The listing builds one solid part. Answer for the finished solid, in the listing's coordinates (mm). Round coordinates to 2 decimals unless told otherwise and drop trailing zeros. Order: outer loops, then holes, each group sorted by start corner. A loop starts at its lowest first (then second) coordinate and runs counter-clockwise, first axis right, second up. Notation, with made-up numbers: M 61.5,48.5 L 76.5,48.5 A10 cw 76.5,58.5 Z; hole C 1,68.5 d3. An arc over 180 degrees is marked long. Write item = value, one per line. Start each with the question number.
(1) Straight lines are drawn through the part: probe 1 along X at (y, z) = (-0.9, 0); probe 2 along X at (y, z) = (-0.65, -30); probe 3 along Y at (x, z) = (-60.6, 0). For each, find the intervals that lie inside material, in ascending order. Write a range as from..to.
(2) A cutting plane is placed at A-A, the plane z = 0. Count the separate pieces of the cut face and the enclosed holes in it, and give its area (3 significant figures).
(3) A cutting plane is placed at B-B, the plane x = -143. Determine the outline of the cut face in (y, z).
(4) Each of these flat-tipped pins is pushed along its axis until it touches: pin 1 (1 mm diameter, centred on x = -60.5, z = 47.5, fed in from -Y); pin 2 (4 mm diameter, centred on y = -8, z = 11, fed in from +X); pin 3 (3.5 mm diameter, centred on x = -16.5, z = -59.5, fed in from -Y). Where does it stop, or does it pass through?
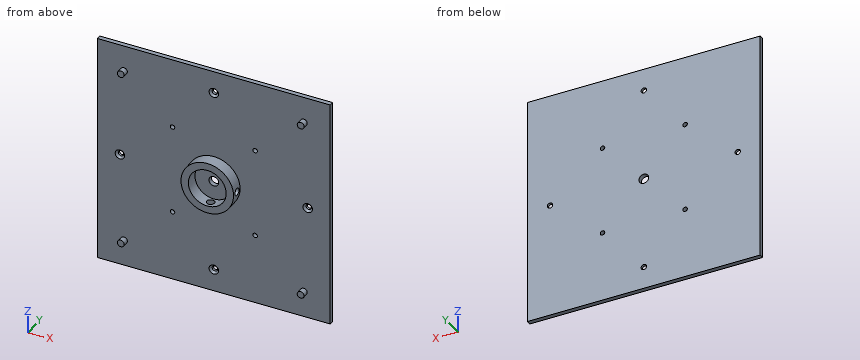
from build123d import *

# Parameters (mm, degrees)
SKETCH10_W                                     = 155
SKETCH10_H                                     = 155
BOSS_EXTRUDE3_DEPTH                            = 3
SKETCH11_R                                     = 17.5
SKETCH11_R_2                                   = 12.59
BOSS_EXTRUDE4_DEPTH                            = 8.4
SKETCH11_4_R                                   = 2.3
BOSS_EXTRUDE6_DEPTH                            = 4
SKETCH12_R                                     = 2.55
CUT_EXTRUDE1_DEPTH                             = 37
SKETCH14_R                                     = 2.55
CUT_EXTRUDE2_DEPTH                             = 75
SKETCH15_R                                     = 1.5
SKETCH15_R_2                                   = 3.25
CUT_EXTRUDE3_DEPTH                             = 95
CSK_FOR_M3_FLAT_HEAD_MACHINE_SCREW1_AT_2_COUNT = 2
CSK_FOR_M3_FLAT_HEAD_MACHINE_SCREW1_AT_2_PITCH = 88.388347648
CSK_FOR_M3_FLAT_HEAD_MACHINE_SCREW1_AT_3_COUNT = 2
CSK_FOR_M3_FLAT_HEAD_MACHINE_SCREW1_AT_3_PITCH = 125
CSK_FOR_M3_FLAT_HEAD_MACHINE_SCREW1_AT_4_COUNT = 2
CSK_FOR_M3_FLAT_HEAD_MACHINE_SCREW1_AT_4_PITCH = 88.388347648


with BuildPart() as part:
    # Sketch10 → Boss-Extrude3 (new body)
    with BuildSketch(Plane.XZ):
        with Locations((-75.370825338, 0)):
            Rectangle(SKETCH10_W, SKETCH10_H)
    extrude(amount=BOSS_EXTRUDE3_DEPTH)

    # Sketch11 → Boss-Extrude4 (add)
    with BuildSketch(Plane.XZ.offset(3)):
        with Locations(Location((-75.370825338, 0, 0), (0, 0, 270))):
            Circle(SKETCH11_R)
        with Locations(Location((-75.370825338, 0, 0), (0, 0, 270))):
            Circle(SKETCH11_R_2, mode=Mode.SUBTRACT)
    extrude(amount=BOSS_EXTRUDE4_DEPTH)

    # Sketch11_4 → Boss-Extrude6 (add)
    with BuildSketch(Plane.XZ.offset(3)):
        with Locations(Location((-135.260825338, 59.89, 0), (0, 0, 90))):
            Circle(SKETCH11_4_R)
        with Locations(Location((-15.480825338, 59.89, 0), (0, 0, 270))):
            Circle(SKETCH11_4_R)
        with Locations(Location((-135.260825338, -59.89, 0), (0, 0, 270))):
            Circle(SKETCH11_4_R)
        with Locations(Location((-15.480825338, -59.89, 0), (0, 0, 90))):
            Circle(SKETCH11_4_R)
    extrude(amount=BOSS_EXTRUDE6_DEPTH)

    # Sketch12 → Cut-Extrude1 (cut)
    with BuildSketch(Plane.XY):
        with Locations((-75.370825338, -6.9)):
            Circle(SKETCH12_R)
    extrude(amount=-CUT_EXTRUDE1_DEPTH, mode=Mode.SUBTRACT)

    # Sketch14 → Cut-Extrude2 (cut)
    with BuildSketch(Plane(origin=(0, 0, 0), x_dir=(0, 0, -1), z_dir=(1, 0, 0))):
        with Locations((0, -6.9)):
            Circle(SKETCH14_R)
    extrude(amount=-CUT_EXTRUDE2_DEPTH, mode=Mode.SUBTRACT)

    # Sketch15 → Cut-Extrude3 (cut)
    with BuildSketch(Plane(origin=(0, 0, 0), x_dir=(1, 0, 0), z_dir=(0, 1, 0))):
        with Locations(Location((-102.870825338, 30, 0), (0, 0, 270))):
            Circle(SKETCH15_R)
        with Locations(Location((-47.870825338, 30, 0), (0, 0, 270))):
            Circle(SKETCH15_R)
        with Locations(Location((-47.870825338, -30, 0), (0, 0, 270))):
            Circle(SKETCH15_R)
        with Locations(Location((-102.870825338, -30, 0), (0, 0, 270))):
            Circle(SKETCH15_R)
        with Locations(Location((-75.370825338, 0, 0), (0, 0, 270))):
            Circle(SKETCH15_R_2)
    extrude(amount=-CUT_EXTRUDE3_DEPTH, mode=Mode.SUBTRACT)

    # Sketch18 → CSK for M3 Flat Head Machine Screw1 (revolve, cut)
    with BuildSketch(Plane(origin=(-75.370825338, -3, -62.5), x_dir=(0, 0, -1), z_dir=(1, 0, 0))):
        Polygon((0, 0), (0, 3), (1.8, 3), (1.8, 1.35), (3.15, 0), align=None)
    csk_for_m3_flat_head_machine_screw1 = revolve(axis=Axis((-75.370825338, -9.35, -62.5), (0, 1, 0)), mode=Mode.SUBTRACT)

    # CSK for M3 Flat Head Machine Screw1 at 2: CSK for M3 Flat Head Machine Screw1 ×2
    with Locations(*[Vector(0.7071067811865477, 0, 0.7071067811865474) * (i * CSK_FOR_M3_FLAT_HEAD_MACHINE_SCREW1_AT_2_PITCH) for i in range(1, CSK_FOR_M3_FLAT_HEAD_MACHINE_SCREW1_AT_2_COUNT)]):
        add(csk_for_m3_flat_head_machine_screw1, mode=Mode.SUBTRACT)

    # CSK for M3 Flat Head Machine Screw1 at 3: CSK for M3 Flat Head Machine Screw1 ×2
    with Locations(*[(0, 0, i * CSK_FOR_M3_FLAT_HEAD_MACHINE_SCREW1_AT_3_PITCH) for i in range(1, CSK_FOR_M3_FLAT_HEAD_MACHINE_SCREW1_AT_3_COUNT)]):
        add(csk_for_m3_flat_head_machine_screw1, mode=Mode.SUBTRACT)

    # CSK for M3 Flat Head Machine Screw1 at 4: CSK for M3 Flat Head Machine Screw1 ×2
    with Locations(*[Vector(-0.7071067811865479, 0, 0.7071067811865472) * (i * CSK_FOR_M3_FLAT_HEAD_MACHINE_SCREW1_AT_4_PITCH) for i in range(1, CSK_FOR_M3_FLAT_HEAD_MACHINE_SCREW1_AT_4_COUNT)]):
        add(csk_for_m3_flat_head_machine_screw1, mode=Mode.SUBTRACT)


solid = part.part
Reported:
q1.probe_1 = -152.87..-139.67, -136.07..-78.62, -72.12..-14.67, -11.07..2.13
q1.probe_2 = -152.87..-104.37, -101.37..-49.37, -46.37..2.13
q1.probe_3 = -11.4..-9.45, -4.35..0
q2.separate_pieces = 5
q2.enclosed_holes = 0
q2.area = 478 mm²
q3.outline = M -3,-77.5 L 0,-77.5 L 0,77.5 L -3,77.5 Z
q4.pin_1 = -3
q4.pin_2 = -60.36
q4.pin_3 = -7
